Here's how the part is built. I have some questions about the finished solid (model axes, mm). Face numbers are marked on the shaded views. A direction names the side the tool comes from. Round coordinates to 2 decimals unless told otherwise and drop trailing zeros. Write each loop counter-clockwise with the first axis right and the second up, starting at its lowest first coordinate (ties: lowest second). Pieces come first, ordered by that corner, then holes. Notation, with made-up numbers: (61, -29.5) - (111, -29.5) arc R22 cw to (111, 7.5) - close; hole circle Ø6 at (-17.5, 60). An arc over 180 degrees is marked (long way). Return JSON: item names as keys, results as strings. Group by question number.
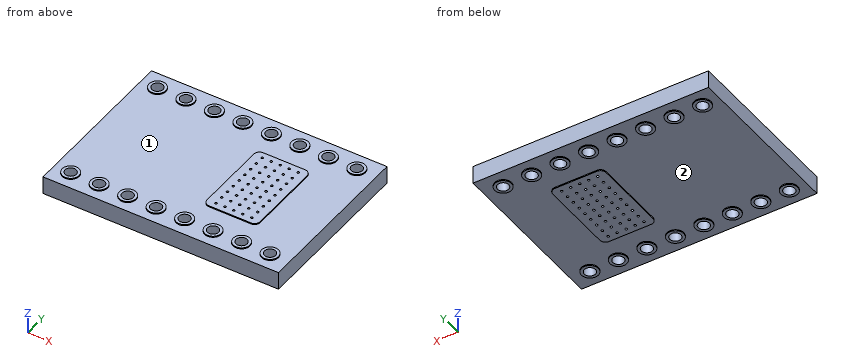
```python
from build123d import *

# Parameters (mm, degrees)
SKETCH1_W                = 21
SKETCH1_H                = 15
BOSS_EXTRUDE1_DEPTH      = 1.6
BOSS_EXTRUDE2_DEPTH      = 0.1
BOSS_EXTRUDE2_DEPTH_BACK = 1.7
SKETCH2_R                = 0.75
SKETCH3_R                = 0.5
CUT_EXTRUDE1_DEPTH       = 2
BOSS_EXTRUDE3_DEPTH      = 0.1
BOSS_EXTRUDE3_DEPTH_BACK = 1.7
SKETCH5_R                = 0.1
CUT_EXTRUDE2_DEPTH       = 1.8


with BuildPart() as part:
    # Sketch1 → Boss-Extrude1 (new body)
    with BuildSketch(Plane.XY):
        Rectangle(SKETCH1_W, SKETCH1_H)
    extrude(amount=BOSS_EXTRUDE1_DEPTH)

    # Sketch2 → Boss-Extrude2 (add, two sides: drawn at the far end of the back side and taken through both)
    with BuildSketch(Plane.XY.offset(1.6).offset(-BOSS_EXTRUDE2_DEPTH_BACK)):
        with Locations((-9, 6)):
            Circle(SKETCH2_R)
        with Locations((-9, -6)):
            Circle(SKETCH2_R)
        with Locations((-6.46, 6)):
            Circle(SKETCH2_R)
        with Locations((-6.46, -6)):
            Circle(SKETCH2_R)
        with Locations((-3.92, 6)):
            Circle(SKETCH2_R)
        with Locations((-3.92, -6)):
            Circle(SKETCH2_R)
        with Locations((-1.38, 6)):
            Circle(SKETCH2_R)
        with Locations((-1.38, -6)):
            Circle(SKETCH2_R)
        with Locations((1.16, 6)):
            Circle(SKETCH2_R)
        with Locations((1.16, -6)):
            Circle(SKETCH2_R)
        with Locations((3.7, 6)):
            Circle(SKETCH2_R)
        with Locations((3.7, -6)):
            Circle(SKETCH2_R)
        with Locations((6.24, 6)):
            Circle(SKETCH2_R)
        with Locations((6.24, -6)):
            Circle(SKETCH2_R)
        with Locations((8.78, 6)):
            Circle(SKETCH2_R)
        with Locations((8.78, -6)):
            Circle(SKETCH2_R)
    extrude(amount=BOSS_EXTRUDE2_DEPTH + BOSS_EXTRUDE2_DEPTH_BACK)

    # Sketch3 → Cut-Extrude1 (cut)
    with BuildSketch(Plane.XY.offset(1.7)):
        with Locations((-9, 6)):
            Circle(SKETCH3_R)
        with Locations((-9, -6)):
            Circle(SKETCH3_R)
        with Locations((-6.46, 6)):
            Circle(SKETCH3_R)
        with Locations((-6.46, -6)):
            Circle(SKETCH3_R)
        with Locations((-3.92, 6)):
            Circle(SKETCH3_R)
        with Locations((-3.92, -6)):
            Circle(SKETCH3_R)
        with Locations((-1.38, 6)):
            Circle(SKETCH3_R)
        with Locations((-1.38, -6)):
            Circle(SKETCH3_R)
        with Locations((1.16, 6)):
            Circle(SKETCH3_R)
        with Locations((1.16, -6)):
            Circle(SKETCH3_R)
        with Locations((3.7, 6)):
            Circle(SKETCH3_R)
        with Locations((3.7, -6)):
            Circle(SKETCH3_R)
        with Locations((6.24, 6)):
            Circle(SKETCH3_R)
        with Locations((6.24, -6)):
            Circle(SKETCH3_R)
        with Locations((8.78, 6)):
            Circle(SKETCH3_R)
        with Locations((8.78, -6)):
            Circle(SKETCH3_R)
    extrude(amount=-CUT_EXTRUDE1_DEPTH, mode=Mode.SUBTRACT)

    # Sketch4 → Boss-Extrude3 (add, two sides: drawn at the far end of the back side and taken through both)
    with BuildSketch(Plane(origin=(0, 0, 0), x_dir=(-1, 0, 0), z_dir=(0, 0, -1)).offset(-BOSS_EXTRUDE3_DEPTH_BACK)):
        with BuildLine():
            Line((-5.625, 3.75), (-1.875, 3.75))
            ThreePointArc((-1.875, 3.75), (-1.521446609, 3.603553391), (-1.375, 3.25))
            Line((-1.375, 3.25), (-1.375, -3.25))
            ThreePointArc((-1.375, -3.25), (-1.521446609, -3.603553391), (-1.875, -3.75))
            Line((-1.875, -3.75), (-5.625, -3.75))
            ThreePointArc((-5.625, -3.75), (-5.978553391, -3.603553391), (-6.125, -3.25))
            Line((-6.125, -3.25), (-6.125, 3.25))
            ThreePointArc((-6.125, 3.25), (-5.978553391, 3.603553391), (-5.625, 3.75))
        make_face()
    extrude(amount=BOSS_EXTRUDE3_DEPTH + BOSS_EXTRUDE3_DEPTH_BACK)

    # Sketch5 → Cut-Extrude2 (cut)
    with BuildSketch(Plane(origin=(0, 0, -0.1), x_dir=(-1, 0, 0), z_dir=(0, 0, -1))):
        with Locations((-3.75, 0)):
            Circle(SKETCH5_R)
        with Locations((-2.95, 0)):
            Circle(SKETCH5_R)
        with Locations((-2.15, 0)):
            Circle(SKETCH5_R)
        with Locations((-4.55, 0)):
            Circle(SKETCH5_R)
        with Locations((-5.35, 0)):
            Circle(SKETCH5_R)
        with Locations((-3.75, -0.8)):
            Circle(SKETCH5_R)
        with Locations((-4.55, -0.8)):
            Circle(SKETCH5_R)
        with Locations((-5.35, -0.8)):
            Circle(SKETCH5_R)
        with Locations((-2.95, -0.8)):
            Circle(SKETCH5_R)
        with Locations((-2.15, -0.8)):
            Circle(SKETCH5_R)
        with Locations((-3.75, -1.6)):
            Circle(SKETCH5_R)
        with Locations((-4.55, -1.6)):
            Circle(SKETCH5_R)
        with Locations((-5.35, -1.6)):
            Circle(SKETCH5_R)
        with Locations((-2.95, -1.6)):
            Circle(SKETCH5_R)
        with Locations((-2.15, -1.6)):
            Circle(SKETCH5_R)
        with Locations((-3.75, -2.4)):
            Circle(SKETCH5_R)
        with Locations((-4.55, -2.4)):
            Circle(SKETCH5_R)
        with Locations((-5.35, -2.4)):
            Circle(SKETCH5_R)
        with Locations((-2.95, -2.4)):
            Circle(SKETCH5_R)
        with Locations((-2.15, -2.4)):
            Circle(SKETCH5_R)
        with Locations((-3.75, -3.2)):
            Circle(SKETCH5_R)
        with Locations((-4.55, -3.2)):
            Circle(SKETCH5_R)
        with Locations((-5.35, -3.2)):
            Circle(SKETCH5_R)
        with Locations((-2.95, -3.2)):
            Circle(SKETCH5_R)
        with Locations((-2.15, -3.2)):
            Circle(SKETCH5_R)
        with Locations((-3.75, 0.8)):
            Circle(SKETCH5_R)
        with Locations((-4.55, 0.8)):
            Circle(SKETCH5_R)
        with Locations((-5.35, 0.8)):
            Circle(SKETCH5_R)
        with Locations((-2.95, 0.8)):
            Circle(SKETCH5_R)
        with Locations((-2.15, 0.8)):
            Circle(SKETCH5_R)
        with Locations((-3.75, 1.6)):
            Circle(SKETCH5_R)
        with Locations((-4.55, 1.6)):
            Circle(SKETCH5_R)
        with Locations((-5.35, 1.6)):
            Circle(SKETCH5_R)
        with Locations((-2.95, 1.6)):
            Circle(SKETCH5_R)
        with Locations((-2.15, 1.6)):
            Circle(SKETCH5_R)
        with Locations((-3.75, 2.4)):
            Circle(SKETCH5_R)
        with Locations((-4.55, 2.4)):
            Circle(SKETCH5_R)
        with Locations((-5.35, 2.4)):
            Circle(SKETCH5_R)
        with Locations((-2.95, 2.4)):
            Circle(SKETCH5_R)
        with Locations((-2.15, 2.4)):
            Circle(SKETCH5_R)
        with Locations((-3.75, 3.2)):
            Circle(SKETCH5_R)
        with Locations((-4.55, 3.2)):
            Circle(SKETCH5_R)
        with Locations((-5.35, 3.2)):
            Circle(SKETCH5_R)
        with Locations((-2.95, 3.2)):
            Circle(SKETCH5_R)
        with Locations((-2.15, 3.2)):
            Circle(SKETCH5_R)
    extrude(amount=-CUT_EXTRUDE2_DEPTH, mode=Mode.SUBTRACT)


solid = part.part
```
1) I need wall thicknesses on line 1 along Y through (x, z) = (8.78, 0.65); line 2 along Y through (x, z) = (-3.5, 0.65); line 3 along Z through (x, y) = (-6, 2). Which ranges of each line are inside material? Lowest first, please.
2) Imagine slicing it at A-A (x = -1.38). Please give me the cut outline in (y, z).
3) Will these pins go through, and if not, where does the flat tip stop? pin 1 Ø2 at (x, y) = (-6.5, -4) entering from +Z; pin 2 Ø4 at (x, y) = (-1, 2) entering from -Z.
4) Imagine slicing it at B-B (z = 0.35). Give the number of separate pieces and of enclosed holes in the cut face, plus the area to 3 significant figures.
5) Imagine slicing it at D-D (y = -4.5). Please give me the cut outline in (x, z), plus the area to 3 significant figures.
6) For the marked faces 1 and 2, which set-ups out of +Z, -Z, +X, -X, +Y, -Y let a thin tool reach every point of the face, with its end or its side?
Results found:
{
 "1": {"line 1": "y = -7.5 to -6.5, -5.5 to 5.5, 6.5 to 7.5", "line 2": "y = -7.5 to -6.27, -5.73 to 5.73, 6.27 to 7.5", "line 3": "z = 0 to 1.6"},
 "2": {"outline": "(-7.5, 0) - (-6.75, 0) - (-6.75, -0.1) - (-6.5, -0.1) - (-6.5, 1.7) - (-6.75, 1.7) - (-6.75, 1.6) - (-7.5, 1.6) - close; (-5.5, -0.1) - (-5.25, -0.1) - (-5.25, 0) - (5.25, 0) - (5.25, -0.1) - (5.5, -0.1) - (5.5, 1.7) - (5.25, 1.7) - (5.25, 1.6) - (-5.25, 1.6) - (-5.25, 1.7) - (-5.5, 1.7) - close; (6.5, -0.1) - (6.75, -0.1) - (6.75, 0) - (7.5, 0) - (7.5, 1.6) - (6.75, 1.6) - (6.75, 1.7) - (6.5, 1.7) - close"},
 "3": {"pin 1": "stops at z = 1.6", "pin 2": "stops at z = 0"},
 "4": {"separate pieces": "1", "enclosed holes": "61", "area": "301 mm²"},
 "5": {"outline": "(-10.5, 0) - (10.5, 0) - (10.5, 1.6) - (-10.5, 1.6) - close", "area": "33.6 mm²"},
 "6": {"face 1": "+Z", "face 2": "-Z"}
}
